```python
from build123d import *

# Parameters (mm, degrees)
CHAMFER_1_SIZE  = 0.2
SKETCH_5_R      = 0.3
EXTRUDE_2_DEPTH = 15
SKETCH_6_R      = 0.5
EXTRUDE_1_DEPTH = 40


# Read off the part's stored shape, not the designer's step: 旋转2
with BuildPart() as part:
    # 旋转2 outline → 旋转2 (revolve)
    with BuildSketch(Plane.YX):
        Polygon((3.1, 0), (0, 0), (0, -27), (2, -27), (2.75, -20), (2.9, -10), (3.1, -10), align=None)
    revolve(axis=Axis((0, 0, 0), (1, 0, 0)))

    # 倒角1
    chamfer_1_edges = [part.edges().sort_by_distance(p)[0] for p in [
        (-10, -3.1, 0),
    ]]
    chamfer(chamfer_1_edges, length=CHAMFER_1_SIZE - 0.0001)  # a hair under: the kernel refuses the full size

    # 草图5 → 拉伸2 (add)
    with BuildSketch(Plane(origin=(0, 0, 0), x_dir=(0, 0, -1), z_dir=(1, 0, 0))):
        with Locations(Location((-0.635, 0.635, 0), (0, 0, 270))):
            Circle(SKETCH_5_R)
        with Locations(Location((-0.635, -0.635, 0), (0, 0, 270))):
            Circle(SKETCH_5_R)
        with Locations(Location((0.635, 0.635, 0), (0, 0, 270))):
            Circle(SKETCH_5_R)
        with Locations(Location((0.635, -0.635, 0), (0, 0, 270))):
            Circle(SKETCH_5_R)
    extrude(amount=EXTRUDE_2_DEPTH)

    # 草图6 → Extrude 1 (add)
    with BuildSketch(Plane.ZY.offset(27)):
        with Locations(Location((0, 0, 0), (0, 0, 90))):
            Circle(SKETCH_6_R)
    extrude(amount=EXTRUDE_1_DEPTH)


solid = part.part
```
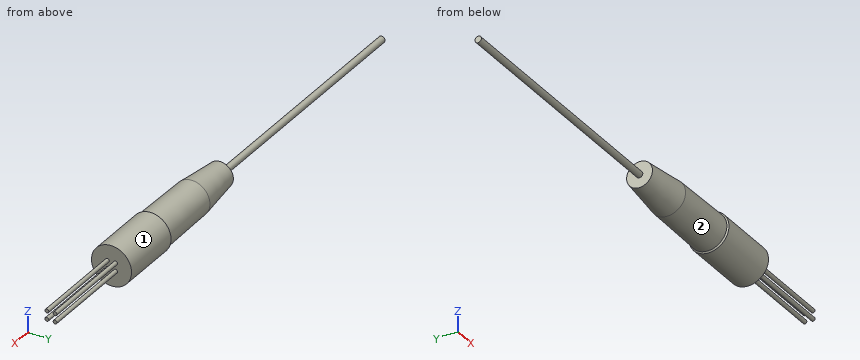
Build history of the part. All positions in model axes, mm. Face numbers are marked on the shaded views. A direction names the side the tool comes from. Round coordinates to 2 decimals unless told otherwise and drop trailing zeros. Loops run counter-clockwise (first coordinate to the right, second up) from the corner with the lowest first, then second, coordinate; pieces in that order, holes last. Notation, with made-up numbers: M 37,8.5 L 75,8.5 A17 ccw 75,30.5 Z; hole C 32,36.25 d8. An arc over 180 degrees is marked long. Answer as CSV lines item,"result".
1. Flat gauge pins, fed straight in: P1, Ø1, axis at x = -7.5, y = -1.5, coming from the +Z side; P2, Ø1, axis at y = -1.5, z = -2, coming from the +X side. Where does each tip first touch, or does it go through?
Resolved:
P1,"stops at z = 2.93"
P2,"stops at x = 0"
2. 3-axis set-ups, long thin cutter, end or side, ignore diameter. For the marked faces 1 and 2: which of +Z, -Z, +X, -X, +Y, -Y reach the whole face in a straight line?
Resolved:
face 1,"+X, -X"
face 2,"-X"
3. Wall check: probe 1 along X at (y, z) = (0, -0.25); probe 2 along X at (y, z) = (-1.75, 0.25); probe 3 along Z at (x, y) = (-23, 1). Give the ranges that are in metal, low to high. Write a range as [from, to].
Resolved:
probe 1,"x = [-67, 0]"
probe 2,"x = [-27, 0]"
probe 3,"z = [-2.21, 2.21]"
4. Cut at B-B on x = -25. Write the cut outline in (y, z), then the cut area to 3 significant figures.
Resolved:
outline,"C 0,0 d4.43"
area,"15.4 mm²"
5. Cut at A-A on x = -4. Write the cut outline in (y, z).
Resolved:
outline,"C 0,0 d6.2"
